from build123d import *

# Parameters (mm, degrees)
ESQUISSE1_R        = 14
ESQUISSE1_R_2      = 1.75
BOSS_EXTRU_1_DEPTH = 17.5
ESQUISSE2_R        = 4.904077813
BOSS_EXTRU_2_DEPTH = 14.25


with BuildPart() as part:
    # Esquisse1 → Boss.-Extru.1 (new body)
    with BuildSketch(Plane.XY):
        Circle(ESQUISSE1_R)
        with Locations((-6.717514421, 6.717514421)):
            Circle(ESQUISSE1_R_2, mode=Mode.SUBTRACT)
        with Locations((6.717514421, 6.717514421)):
            Circle(ESQUISSE1_R_2, mode=Mode.SUBTRACT)
        with Locations((6.717514421, -6.717514421)):
            Circle(ESQUISSE1_R_2, mode=Mode.SUBTRACT)
        with Locations((-6.717514421, -6.717514421)):
            Circle(ESQUISSE1_R_2, mode=Mode.SUBTRACT)
    extrude(amount=BOSS_EXTRU_1_DEPTH)

    # Esquisse2 → Boss.-Extru.2 (add)
    with BuildSketch(Plane(origin=(0, 0, 0), x_dir=(-1, 0, 0), z_dir=(0, 0, -1))):
        with Locations(Location((0, 0, 0), (0, 0, 180))):
            Circle(ESQUISSE2_R)
    extrude(amount=BOSS_EXTRU_2_DEPTH)


solid = part.part
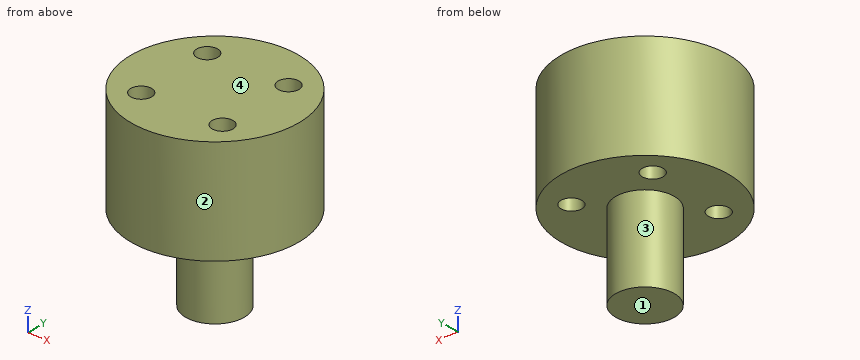
Could you check a few things on this model? Use its own coordinates, in mm. Face numbers are marked on the shaded views. A direction names the side the tool comes from. Coordinates: 2 decimals unless noted, no trailing zeros. Order: outer loops, then holes, each group sorted by start corner. A loop starts at its lowest first (then second) coordinate and runs counter-clockwise, first axis right, second up. Notation, with made-up numbers: (-0.5, 23) -> (43.5, 23) arc R31 cw to (43.5, 61) -> close; hole circle Ø10 at (87.25, 21.5). An arc over 180 degrees is marked (long way). One line per item, written item: value. Start each with the question number.
1) Imagine slicing it at B-B on y = 0. List the corners of the cut face in (x, z) for me.
2) If I drill on L1, parallel to X at y = 5.75, z = 11.5; L2, parallel to Y at x = 6.5, z = 10; L3, parallel to Y at x = -6.25, z = 13, over which ranges is the centre line in solid material (lowest first)? Write a range as [from, to].
3) Imagine slicing it at A-A on x = -5.75. List the corners of the cut face in (y, z) for me, plus the area to 3 significant figures.
4) Which directions (+Z, -Z, +X, -X, +Y, -Y) give clear straight access to the entire face, cutting with the end or side of a thin tool? Please do the marked faces 3 and 4.
5) Imagine slicing it at D-D on z = -10. List the corners of the cut face in (x, y) for me, plus the area to 3 significant figures.
6) I'm going to push flat-ended pins straight in: pin 1 (3 mm diameter, centred on x = 6.72, y = 6.72, fed in from -Z); pin 2 (6 mm diameter, centred on x = 10.5, z = 13.5, fed in from -Y); pin 3 (5 mm diameter, centred on y = 0.5, z = -4, fed in from +X); pin 4 (4.5 mm diameter, centred on x = -6.72, y = 6.72, fed in from -Z). Where does each tip first touch, or does it pass through?
7) We'd pull the mould along Y, two halves only. Please class the marked faces 1 and 2: +Y half, -Y half, draft (parallel to the pull), parting line (faces both ways), or undercut.
Answer list:
1. outline: (-14, 0) -> (-4.9, 0) -> (-4.9, -14.25) -> (4.9, -14.25) -> (4.9, 0) -> (14, 0) -> (14, 17.5) -> (-14, 17.5) -> close
2. L1: x = [-12.76, -8.18], [-5.26, 5.26], [8.18, 12.76]
2. L2: y = [-12.4, -8.45], [-4.98, 4.98], [8.45, 12.4]
2. L3: y = [-12.53, -8.4], [-5.03, 5.03], [8.4, 12.53]
3. outline: (-12.76, 0) -> (-8.18, 0) -> (-8.18, 17.5) -> (-12.76, 17.5) -> close; (-5.26, 0) -> (5.26, 0) -> (5.26, 17.5) -> (-5.26, 17.5) -> close; (8.18, 0) -> (12.76, 0) -> (12.76, 17.5) -> (8.18, 17.5) -> close
3. area: 345 mm2
4. face 3: -Z
4. face 4: +Z, +X, -X, +Y, -Y
5. outline: circle Ø9.81 at (0, 0)
5. area: 75.6 mm2
6. pin 1: passes through
6. pin 2: stops at y = -11.82
6. pin 3: stops at x = 4.9
6. pin 4: stops at z = 0
7. face 1: draft
7. face 2: parting line
